from build123d import *

# Parameters (mm, degrees)
SKETCH1_W                = 76.2
SKETCH1_H                = 63.5
BOSS_EXTRUDE2_DEPTH      = 63.5
SKETCH6_W                = 38.1
SKETCH6_H                = 50.8
CUT_EXTRUDE4_DEPTH       = 63.5
CUT_EXTRUDE6_DEPTH       = 118.774954893
CUT_EXTRUDE6_DEPTH_BACK  = 118.774954893
SKETCH9_R                = 5.08
CUT_EXTRUDE7_DEPTH       = 118.774954893
CUT_EXTRUDE10_DEPTH      = 118.774954893
CUT_EXTRUDE15_DEPTH      = 118.774954893
CUT_EXTRUDE15_DEPTH_BACK = 118.774954893


with BuildPart() as part:
    # Sketch1 → Boss-Extrude2 (new body)
    with BuildSketch(Plane(origin=(0, 0, 0), x_dir=(1, 0, 0), z_dir=(0, 1, 0))):
        with Locations((38.1, 31.75)):
            Rectangle(SKETCH1_W, SKETCH1_H)
    boss_extrude2 = extrude(amount=BOSS_EXTRUDE2_DEPTH)

    # Sketch6 → Cut-Extrude4 (cut)
    with BuildSketch(Plane.XY):
        with Locations((38.1, 38.1)):
            Rectangle(SKETCH6_W, SKETCH6_H)
    cut_extrude4 = extrude(amount=-CUT_EXTRUDE4_DEPTH, mode=Mode.SUBTRACT)

    # Sketch7 → Cut-Extrude6 (cut, two sides: drawn at the far end of the back side and taken through both)
    with BuildSketch(Plane(origin=(0, 0, 0), x_dir=(1, 0, 0), z_dir=(0, 1, 0)).offset(-CUT_EXTRUDE6_DEPTH_BACK)):
        Polygon((38.1, -158.106178129), (38.1, 0), (38.1, 63.5), (38.1, 221.606178129), (354.312356258, 221.606178129), (354.312356258, -158.106178129), align=None)
    extrude(amount=CUT_EXTRUDE6_DEPTH + CUT_EXTRUDE6_DEPTH_BACK, mode=Mode.SUBTRACT)

    # Mirror3: Boss-Extrude2, Cut-Extrude4 across plane
    add(boss_extrude2.mirror(Plane(origin=(38.1, 226.593693616, 0), x_dir=(0, 0, 1), z_dir=(-1, 0, 0))))
    add(cut_extrude4.mirror(Plane(origin=(38.1, 226.593693616, 0), x_dir=(0, 0, 1), z_dir=(-1, 0, 0))), mode=Mode.SUBTRACT)

    # Sketch9 → Cut-Extrude7 (cut, through all)
    with BuildSketch(Plane.ZY):
        with Locations((-31.75, 53.34)):
            Circle(SKETCH9_R)
    extrude(amount=-CUT_EXTRUDE7_DEPTH, mode=Mode.SUBTRACT)

    # Sketch10 → Cut-Extrude10 (cut, through all)
    with BuildSketch(Plane.ZY):
        with BuildLine():
            Line((-63.5, 63.5), (-63.5, 25.4))
            Line((-63.5, 25.4), (-43.307, 58.60552476))
            ThreePointArc((-43.307, 58.60552476), (-41.64587309, 61.300006016), (-39.37, 63.5))
            Line((-39.37, 63.5), (-63.5, 63.5))
        make_face()
        with BuildLine():
            ThreePointArc((-24.13, 63.5), (-21.85412691, 61.300006016), (-20.193, 58.60552476))
            Line((-20.193, 58.60552476), (0, 25.4))
            Line((0, 25.4), (0, 63.5))
            Line((0, 63.5), (-24.13, 63.5))
        make_face()
    extrude(amount=-CUT_EXTRUDE10_DEPTH, mode=Mode.SUBTRACT)

    # Sketch11 → Cut-Extrude15 (cut, two sides: drawn at the far end of the back side and taken through both)
    with BuildSketch(Plane(origin=(0, 0, 0), x_dir=(1, 0, 0), z_dir=(0, 1, 0)).offset(-CUT_EXTRUDE15_DEPTH_BACK)):
        with BuildLine():
            Line((40.64, 50.8), (40.64, 12.7))
            ThreePointArc((40.64, 12.7), (38.1, 10.16), (35.56, 12.7))
            Line((35.56, 12.7), (35.56, 50.8))
            ThreePointArc((35.56, 50.8), (38.1, 53.34), (40.64, 50.8))
        make_face()
    extrude(amount=CUT_EXTRUDE15_DEPTH + CUT_EXTRUDE15_DEPTH_BACK, mode=Mode.SUBTRACT)


solid = part.part
Design review of the part built by this model. Coordinates are the model's own, in mm. A direction names the side the tool comes from. Round coordinates to 2 decimals unless told otherwise and drop trailing zeros. Order: outer loops, then holes, each group sorted by start corner. A loop starts at its lowest first (then second) coordinate and runs counter-clockwise, first axis right, second up.
1) Consider section C-C (x = 38.1). State the section outline as (y, z) points, plus the area to 3 significant figures.
The answers:
outline: (0, -63.5) - (12.7, -63.5) - (12.7, -53.34) - (0, -53.34) - close; (0, -10.16) - (12.7, -10.16) - (12.7, 0) - (0, 0) - close
area: 258 mm2
2) Clearance check with flat-ended pins moving along their axes: pin 1 Ø10 at (y, z) = (46, -56.5) entering from -X; pin 2 Ø19 at (x, z) = (41.5, -42) entering from +Y; pin 3 Ø9 at (y, z) = (53.34, -31.75) entering from -X. State where each tip first meets the part, or that it passes through.
The answers:
pin 1: stops at x = 0
pin 2: stops at y = 12.7
pin 3: passes through
3) Machinability: for faces 1 (the flat face through (57.15, 32, -31)), 2 (the flat face through (67, 63.5, -32)), 3 (the cylindrical face through (38.16, 6.26, -10.16)), which of the approach directions +Z, -Z, +X, -X, +Y, -Y give a long, thin tool a straight path to every point of the face, cutting with its end or side? Answer none if there is none.
The answers:
face 1: +Z, -Z, +Y
face 2: +Z, -Z, +X, -X, +Y
face 3: +Y, -Y
4) Consider section B-B (z = -38). State the section outline as (x, y) points.
The answers:
outline: (0, 0) - (35.56, 0) - (35.56, 12.7) - (19.05, 12.7) - (19.05, 63.5) - (0, 63.5) - close; (40.64, 0) - (76.2, 0) - (76.2, 63.5) - (57.15, 63.5) - (57.15, 12.7) - (40.64, 12.7) - close
5) Consider section A-A (y = 15.5). State the section outline as (x, z) points, plus the area to 3 significant figures.
The answers:
outline: (0, -63.5) - (19.05, -63.5) - (19.05, 0) - (0, 0) - close; (57.15, -63.5) - (76.2, -63.5) - (76.2, 0) - (57.15, 0) - close
area: 2,420 mm2
6) For L1, parallel to X at y = 8.5, z = -33; L2, parallel to X at y = 14.5, z = -51.5; L3, parallel to Y at x = 5.5, z = -31.75, list the stretches that pass through material, from the lowest coordinate up.
The answers:
L1: x = 0 to 35.56, 40.64 to 76.2
L2: x = 0 to 19.05, 57.15 to 76.2
L3: y = 0 to 48.26, 58.42 to 63.5
7) Consider section D-D (x = 66). State the section outline as (y, z) points, plus the area to 3 significant figures.
The answers:
outline: (0, -63.5) - (25.4, -63.5) - (58.61, -43.31) arc R12.7 ccw to (63.5, -39.37) - (63.5, -24.13) arc R12.7 ccw to (58.61, -20.19) - (25.4, 0) - (0, 0) - close; hole circle Ø10.16 at (53.34, -31.75)
area: 3,070 mm2
8) Draft analysis for pull direction Y (two halves, no side actions). For faces 4 (the flat face through (47, 0, -32)), 5 (the flat face through (19.05, 32, -31)), 6 (the cylindrical face through (9.392, 57.623, -29.019)), state which applies: released by +Y, released by -Y, zero draft, split by the parting line, or undercut.
The answers:
face 4: released by -Y
face 5: zero draft
face 6: undercut
